Read the model definition and answer for the solid it produces. Units are mm, in the model's axes. A direction names the side the tool comes from. Coordinates: 2 decimals unless noted, no trailing zeros. Order: outer loops, then holes, each group sorted by start corner. A loop starts at its lowest first (then second) coordinate and runs counter-clockwise, first axis right, second up. Notation, with made-up numbers: M 35.25,83 L 87.25,83 A8 ccw 87.25,98 Z; hole C 31,82 d6. An arc over 180 degrees is marked long. One line per question, with ' | ' between items. Start each with the question number.
1) Find section D-D, the plane x = 7.5. Write down the section's boundary in (y, z).
2) Find section B-B, the plane z = -11. Write down the section's boundary in (x, y).
3) Find section A-A, the plane x = 0. Write down the section's boundary in (y, z).
4) Consider probe 1 along Y at (x, z) = (-0.25, 4.5); probe 2 along Y at (x, z) = (-2.25, -2.75); probe 3 along Y at (x, z) = (9.5, 6.5). Determine where each line is inside the solid, lowest interval first.
5) Find section C-C, the plane y = 53. Write down the section's boundary in (x, z), plus the area to 3 significant figures.
6) The mould has two halves that part along X. Classify faces 5 (the face through (0, 8, 0)), 6 (the face through (-5, 30, 0)), 7 (the face through (6, 0, 3)), 8 (the face through (3.44, 24.64, -2.04)): +X half, -X half, draft (parallel to the pull), parting line (faces both ways), or undercut.
7) A tool of negligible diameter and unlimited length cuts with its end or side. For faces 1 (the face through (4, 34.5, -2)), 2 (the face through (6, 4, 0)), 3 (the face through (-3, 3, -1)), 4 (the face through (0, 25, 4)), from which of +Z, -Z, +X, -X, +Y, -Y can it reach the whole face along a straight path? Write none if from no direction.
8) Given P1, Ø3, axis at x = -11, z = 0.01, coming from the +Y side; P2, Ø12, axis at x = -6, y = 9.5, coming from the +Z side; P3, Ø5, axis at x = -7, y = 50, coming from the +Z side; P4, Ø13, axis at x = 5, z = 2, coming from the +Y side, each flat-ended and moving along its own axis, determine where each tip first touches the part or whether it passes through.
from build123d import *

# Parameters (mm, degrees)
SKETCH_1_R          = 13
EXTRUDE_1_DEPTH     = 4
SKETCH_2_R          = 5
EXTRUDE_2_DEPTH     = 52.5
CUT_EXTRUDE_1_REACH = 6
SKETCH_3_R          = 1.25
SKETCH_4_W          = 6
SKETCH_4_H          = 20
CUT_EXTRUDE_2_DEPTH = 1
SKETCH_5_W          = 20
SKETCH_5_H          = 6
CUT_EXTRUDE_3_DEPTH = 1
SKETCH_6_R          = 6
CUT_EXTRUDE_5_DEPTH = 3
SKETCH_7_R          = 3
CUT_EXTRUDE_6_DEPTH = 5


with BuildPart() as part:
    # 스케치1 → 보스-돌출1 (new body)
    with BuildSketch(Plane(origin=(0, 0, 0), x_dir=(1, 0, 0), z_dir=(0, 1, 0))):
        Circle(SKETCH_1_R)
    extrude(amount=EXTRUDE_1_DEPTH)

    # 스케치2 → 보스-돌출2 (add)
    with BuildSketch(Plane(origin=(0, 4, 0), x_dir=(1, 0, 0), z_dir=(0, 1, 0))):
        Circle(SKETCH_2_R)
    extrude(amount=EXTRUDE_2_DEPTH)

    # 스케치3 → 컷-돌출1 (cut, up to next)
    with BuildSketch(Plane(origin=(0, 4, 0), x_dir=(1, 0, 0), z_dir=(0, 1, 0)), mode=Mode.PRIVATE) as cut_extrude_1_sk1:
        with Locations((0, 11)):
            Circle(SKETCH_3_R)
    cut_extrude_1_tool1 = extrude(cut_extrude_1_sk1.sketch, amount=-CUT_EXTRUDE_1_REACH, mode=Mode.PRIVATE) & part.part
    add(cut_extrude_1_tool1.solids().sort_by_distance((0, 4, -11))[0], mode=Mode.SUBTRACT)
    # 스케치3 → 컷-돌출1 (cut, up to next)
    with BuildSketch(Plane(origin=(0, 4, 0), x_dir=(1, 0, 0), z_dir=(0, 1, 0)), mode=Mode.PRIVATE) as cut_extrude_1_sk2:
        with Locations((7.781876099, 7.779707807)):
            Circle(SKETCH_3_R)
    cut_extrude_1_tool2 = extrude(cut_extrude_1_sk2.sketch, amount=-CUT_EXTRUDE_1_REACH, mode=Mode.PRIVATE) & part.part
    add(cut_extrude_1_tool2.solids().sort_by_distance((7.781876, 4, -7.779708))[0], mode=Mode.SUBTRACT)
    # 스케치3 → 컷-돌출1 (cut, up to next)
    with BuildSketch(Plane(origin=(0, 4, 0), x_dir=(1, 0, 0), z_dir=(0, 1, 0)), mode=Mode.PRIVATE) as cut_extrude_1_sk3:
        with Locations((11.007403012, 0)):
            Circle(SKETCH_3_R)
    cut_extrude_1_tool3 = extrude(cut_extrude_1_sk3.sketch, amount=-CUT_EXTRUDE_1_REACH, mode=Mode.PRIVATE) & part.part
    add(cut_extrude_1_tool3.solids().sort_by_distance((11.007403, 4, 0))[0], mode=Mode.SUBTRACT)
    # 스케치3 → 컷-돌출1 (cut, up to next)
    with BuildSketch(Plane(origin=(0, 4, 0), x_dir=(1, 0, 0), z_dir=(0, 1, 0)), mode=Mode.PRIVATE) as cut_extrude_1_sk4:
        with Locations((7.787110819, -7.781876099)):
            Circle(SKETCH_3_R)
    cut_extrude_1_tool4 = extrude(cut_extrude_1_sk4.sketch, amount=-CUT_EXTRUDE_1_REACH, mode=Mode.PRIVATE) & part.part
    add(cut_extrude_1_tool4.solids().sort_by_distance((7.787111, 4, 7.781876))[0], mode=Mode.SUBTRACT)
    # 스케치3 → 컷-돌출1 (cut, up to next)
    with BuildSketch(Plane(origin=(0, 4, 0), x_dir=(1, 0, 0), z_dir=(0, 1, 0)), mode=Mode.PRIVATE) as cut_extrude_1_sk5:
        with Locations((0.007403012, -11.007403012)):
            Circle(SKETCH_3_R)
    cut_extrude_1_tool5 = extrude(cut_extrude_1_sk5.sketch, amount=-CUT_EXTRUDE_1_REACH, mode=Mode.PRIVATE) & part.part
    add(cut_extrude_1_tool5.solids().sort_by_distance((0.007403, 4, 11.007403))[0], mode=Mode.SUBTRACT)
    # 스케치3 → 컷-돌출1 (cut, up to next)
    with BuildSketch(Plane(origin=(0, 4, 0), x_dir=(1, 0, 0), z_dir=(0, 1, 0)), mode=Mode.PRIVATE) as cut_extrude_1_sk6:
        with Locations((-7.774473087, -7.787110819)):
            Circle(SKETCH_3_R)
    cut_extrude_1_tool6 = extrude(cut_extrude_1_sk6.sketch, amount=-CUT_EXTRUDE_1_REACH, mode=Mode.PRIVATE) & part.part
    add(cut_extrude_1_tool6.solids().sort_by_distance((-7.774473, 4, 7.787111))[0], mode=Mode.SUBTRACT)
    # 스케치3 → 컷-돌출1 (cut, up to next)
    with BuildSketch(Plane(origin=(0, 4, 0), x_dir=(1, 0, 0), z_dir=(0, 1, 0)), mode=Mode.PRIVATE) as cut_extrude_1_sk7:
        with Locations((-11, -0.007403012)):
            Circle(SKETCH_3_R)
    cut_extrude_1_tool7 = extrude(cut_extrude_1_sk7.sketch, amount=-CUT_EXTRUDE_1_REACH, mode=Mode.PRIVATE) & part.part
    add(cut_extrude_1_tool7.solids().sort_by_distance((-11, 4, 0.007403))[0], mode=Mode.SUBTRACT)
    # 스케치3 → 컷-돌출1 (cut, up to next)
    with BuildSketch(Plane(origin=(0, 4, 0), x_dir=(1, 0, 0), z_dir=(0, 1, 0)), mode=Mode.PRIVATE) as cut_extrude_1_sk8:
        with Locations((-7.779707807, 7.774473087)):
            Circle(SKETCH_3_R)
    cut_extrude_1_tool8 = extrude(cut_extrude_1_sk8.sketch, amount=-CUT_EXTRUDE_1_REACH, mode=Mode.PRIVATE) & part.part
    add(cut_extrude_1_tool8.solids().sort_by_distance((-7.779708, 4, -7.774473))[0], mode=Mode.SUBTRACT)

    # 스케치4 → 컷-돌출2 (cut)
    with BuildSketch(Plane.XY.offset(5)):
        with Locations((0, 24.5)):
            Rectangle(SKETCH_4_W, SKETCH_4_H)
    extrude(amount=-CUT_EXTRUDE_2_DEPTH, mode=Mode.SUBTRACT)

    # 스케치5 → 컷-돌출3 (cut)
    with BuildSketch(Plane(origin=(4.330127019, 0, -2.5), x_dir=(0, -1, 0), z_dir=(0.866025404, 0, -0.5))):
        with Locations((-24.5, 0)):
            Rectangle(SKETCH_5_W, SKETCH_5_H)
    extrude(amount=-CUT_EXTRUDE_3_DEPTH, mode=Mode.SUBTRACT)

    # 스케치6 → 컷-돌출5 (cut)
    with BuildSketch(Plane.XZ):
        Circle(SKETCH_6_R)
    extrude(amount=-CUT_EXTRUDE_5_DEPTH, mode=Mode.SUBTRACT)

    # 스케치7 → 컷-돌출6 (cut)
    with BuildSketch(Plane.XZ.offset(-3)):
        Circle(SKETCH_7_R)
    extrude(amount=-CUT_EXTRUDE_6_DEPTH, mode=Mode.SUBTRACT)


solid = part.part
Report:
1) outline: M 0,-10.62 L 4,-10.62 L 4,-9 L 0,-9 Z; M 0,-6.56 L 4,-6.56 L 4,6.57 L 0,6.57 Z; M 0,9 L 4,9 L 4,10.62 L 0,10.62 Z
2) outline: M -6.93,0 L -1.25,0 L -1.25,4 L -6.93,4 Z; M 1.25,0 L 6.93,0 L 6.93,4 L 1.25,4 Z
3) outline: M 0,-13 L 4,-13 L 4,-12.25 L 0,-12.25 Z; M 0,-9.75 L 4,-9.75 L 4,-5 L 56.5,-5 L 56.5,5 L 34.5,5 L 34.5,4 L 14.5,4 L 14.5,5 L 4,5 L 4,9.76 L 0,9.76 L 0,6 L 3,6 L 3,3 L 8,3 L 8,-3 L 3,-3 L 3,-6 L 0,-6 Z; M 0,12.26 L 4,12.26 L 4,13 L 0,13 Z
4) probe 1: y = 3 to 14.5, 34.5 to 56.5 | probe 2: y = 3 to 56.5 | probe 3: y = 0 to 4
5) outline: C 0,0 d10 | area: 78.5 mm^2
6) face 5: undercut | face 6: parting line | face 7: draft | face 8: +X half
7) face 1: -Z, +X | face 2: +Y | face 3: -Y | face 4: +Z, +X, -X
8) P1: stops at y = 4 | P2: stops at z = 12.49 | P3: stops at z = 2.18 | P4: stops at y = 56.5
